Here's how the part is built. I have some questions about the finished solid (model axes, mm). Face numbers are marked on the shaded views. Coordinates: 2 decimals unless noted, no trailing zeros. Write each loop counter-clockwise with the first axis right and the second up, starting at its lowest first coordinate (ties: lowest second). Pieces come first, ordered by that corner, then holes.
Item 1: Please list where these lines run through material, in increasing order: line 1 (Z direction, x = 0.25, y = 2.25); line 2 (Z direction, x = 0.4, y = 2.5); line 3 (Z direction, x = 0.1, y = 1.25).
Item 2: If we mould it in two halves opening along Z, with no side actions, what happens to the marked faces 1, 2 and 3? For each: pulls with the +Z half, pulls with the -Z half, needs draft (parallel to the pull), parting line crosses it, or undercut.
Item 3: I'm going to push a flat-ended pin straight in: P1, Ø3, axis at y = 1, z = -1.5, coming from the -X side. Where does the tip first touch, or does it pass through?
Item 4: I want a section at D-D (z = 0). Please give me the cut outline in (x, y).
Item 5: I want a section at A-A (x = 0.5). Please give me the cut outline in (y, z), and give its area (3 significant figures).
Item 6: I want a section at B-B (y = 2.25). Please give me the cut outline in (x, z).
Item 7: I want a section at C-C (z = 3). Please give me the cut outline in (x, y), and give its area (3 significant figures).
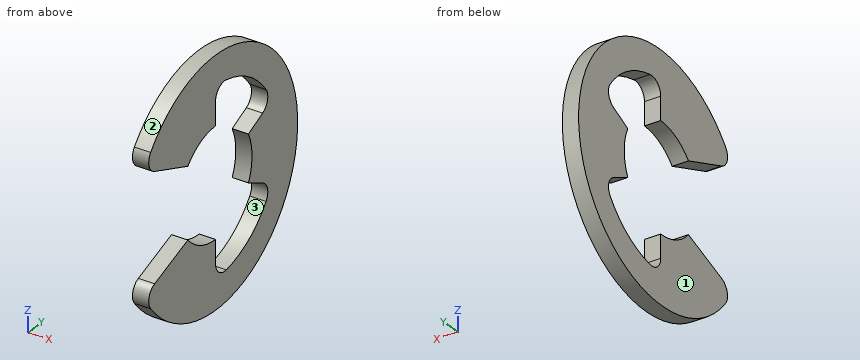
from build123d import *

# Parameters (mm, degrees)
BOSS_EXTRUDE1_DEPTH = 0.6


with BuildPart() as part:
    # Sketch1 → Boss-Extrude1 (new body)
    with BuildSketch(Plane(origin=(0, 0, 0), x_dir=(0, 0, -1), z_dir=(1, 0, 0))):
        with BuildLine():
            Line((2.856571371, 0), (2, 0))
            ThreePointArc((2, 0), (1.816590212, -0.836660027), (1.3, -1.519868415))
            Line((1.3, -1.519868415), (1.979902452, -3.338350127))
            ThreePointArc((1.979902452, -3.338350127), (2.311420831, -3.644163179), (2.754268365, -3.558652241))
            ThreePointArc((2.754268365, -3.558652241), (0, 4.5), (-2.754268365, -3.558652241))
            ThreePointArc((-2.754268365, -3.558652241), (-2.311420831, -3.644163179), (-1.979902452, -3.338350127))
            Line((-1.979902452, -3.338350127), (-1.3, -1.519868415))
            ThreePointArc((-1.3, -1.519868415), (-1.816590212, -0.836660027), (-2, 0))
            Line((-2, 0), (-2.856571371, 0))
            ThreePointArc((-2.856571371, 0), (-3.239392118, 0.17836624), (-3.349083677, 0.586206897))
            ThreePointArc((-3.349083677, 0.586206897), (-2.875474594, 1.814289354), (-1.970919405, 2.770465069))
            ThreePointArc((-1.970919405, 2.770465069), (-1.555584997, 2.847039011), (-1.229785674, 2.578299284))
            Line((-1.229785674, 2.578299284), (-0.861022194, 1.805170569))
            ThreePointArc((-0.861022194, 1.805170569), (0, 2), (0.861022194, 1.805170569))
            Line((0.861022194, 1.805170569), (1.229785674, 2.578299284))
            ThreePointArc((1.229785674, 2.578299284), (1.555584997, 2.847039011), (1.970919405, 2.770465069))
            ThreePointArc((1.970919405, 2.770465069), (2.875474594, 1.814289354), (3.349083677, 0.586206897))
            ThreePointArc((3.349083677, 0.586206897), (3.239392118, 0.17836624), (2.856571371, 0))
        make_face()
    extrude(amount=BOSS_EXTRUDE1_DEPTH)


solid = part.part
Answer:
1. line 1: z = -3.9 to -2.55, -1.07 to 1.07, 2.55 to 3.9
1. line 2: z = -3.74 to -2.3, -1.19 to 1.19, 2.3 to 3.74
1. line 3: z = -4.32 to -3.16, 3.16 to 4.32
2. face 1: needs draft
2. face 2: parting line crosses it
2. face 3: undercut
3. P1: stops at x = 0
4. outline: (0, 2) - (0.6, 2) - (0.6, 4.5) - (0, 4.5) - close
5. outline: (-3.56, -2.75) arc R4.5 ccw (long way) to (-3.56, 2.75) arc R0.5 ccw to (-3.34, 1.98) - (-1.52, 1.3) arc R2 cw to (0, 2) - (0, 2.86) arc R0.5 cw to (0.59, 3.35) arc R3.4 cw to (2.77, 1.97) arc R0.5 cw to (2.58, 1.23) - (1.81, 0.86) arc R2 cw to (1.81, -0.86) - (2.58, -1.23) arc R0.5 cw to (2.77, -1.97) arc R3.4 cw to (0.59, -3.35) arc R0.5 cw to (0, -2.86) - (0, -2) arc R2 cw to (-1.52, -1.3) - (-3.34, -1.98) arc R0.5 ccw to start
5. area: 33.4 mm2
6. outline: (0, -3.9) - (0.6, -3.9) - (0.6, -2.55) - (0, -2.55) - close; (0, -1.07) - (0.6, -1.07) - (0.6, 1.07) - (0, 1.07) - close; (0, 2.55) - (0.6, 2.55) - (0.6, 3.9) - (0, 3.9) - close
7. outline: (0, -3.35) - (0.6, -3.35) - (0.6, 0.02) - (0, 0.02) - close; (0, 1.6) - (0.6, 1.6) - (0.6, 3.35) - (0, 3.35) - close
7. area: 3.08 mm2
